```python
from build123d import *

# Parameters (mm, degrees)
BOSS_EXTRUDE1_DEPTH = 50.8
SKETCH2_R           = 2.667
CUT_EXTRUDE1_DEPTH  = 3.175
SKETCH3_R           = 2.667
CUT_EXTRUDE2_DEPTH  = 3.175
FILLET1_R           = 2.159


with BuildPart() as part:
    # Sketch1 → Boss-Extrude1 (new body)
    with BuildSketch(Plane(origin=(0, 0, 0), x_dir=(0, 0, -1), z_dir=(1, 0, 0))):
        Polygon((0, 0), (0, 25.4), (-3.175, 25.4), (-3.175, 3.175), (-25.4, 3.175), (-25.4, 0), align=None)
    extrude(amount=BOSS_EXTRUDE1_DEPTH)

    # Sketch2 → Cut-Extrude1 (cut)
    with BuildSketch(Plane(origin=(0, 3.175, 0), x_dir=(1, 0, 0), z_dir=(0, 1, 0))):
        with Locations((11.938, -19.05)):
            Circle(SKETCH2_R)
        with Locations((37.338, -19.05)):
            Circle(SKETCH2_R)
    extrude(amount=-CUT_EXTRUDE1_DEPTH, mode=Mode.SUBTRACT)

    # Sketch3 → Cut-Extrude2 (cut)
    with BuildSketch(Plane.XY.offset(3.175)):
        with Locations((38.1, 14.351)):
            Circle(SKETCH3_R)
        with Locations((12.7, 14.351)):
            Circle(SKETCH3_R)
    extrude(amount=-CUT_EXTRUDE2_DEPTH, mode=Mode.SUBTRACT)

    # Fillet1
    fillet1_edges = [part.edges().sort_by_distance(p)[0] for p in [
        (25.4, 3.175, 3.175),
        (25.4, 0, 0),
    ]]
    fillet(fillet1_edges, radius=FILLET1_R)


solid = part.part
```
Geometry: final body of the model. Coordinates: model frame, mm. A direction names the side the tool comes from. Round coordinates to 2 decimals unless told otherwise and drop trailing zeros. Loops run counter-clockwise (first coordinate to the right, second up) from the corner with the lowest first, then second, coordinate; pieces in that order, holes last.
Item 1: Mould query, pull axis Y, two halves, no side actions, for faces 1 (the flat face through (0, 2, 6)), 2 (the flat face through (25, 0, 14)), 3 (the cylindrical face through (36.13, 16.15, 1.61)). Classes: released by +Y, released by -Y, zero draft, split by the parting line, or undercut.
Checked values:
face 1: zero draft
face 2: released by -Y
face 3: undercut
Item 2: Contact query for flat-ended pins moving along their axis: P1, Ø5, axis at x = 12.7, y = 14.351, coming from the -Z side; P2, Ø8.5, axis at x = 37.338, z = 19.05, coming from the +Y side (3 decimals); P3, Ø5, axis at x = 38.5, y = 17, coming from the +Z side (3 decimals). Output: stop coordinate, or through.
Checked values:
P1: passes through
P2: stops at y = 3.175
P3: stops at z = 3.175
Item 3: Section A-A, the plane z = 19.05. Output: boundary loops of the cut face in (x, y) (3 decimals).
Checked values:
outline: (0, 0) - (9.271, 0) - (9.271, 3.175) - (0, 3.175) - close; (14.605, 0) - (34.671, 0) - (34.671, 3.175) - (14.605, 3.175) - close; (40.005, 0) - (50.8, 0) - (50.8, 3.175) - (40.005, 3.175) - close
Item 4: Section D-D, the plane x = 25.5. Output: boundary loops of the cut face in (y, z) (3 decimals).
Checked values:
outline: (0, 2.159) arc R2.159 ccw to (2.159, 0) - (25.4, 0) - (25.4, 3.175) - (5.334, 3.175) arc R2.159 cw to (3.175, 5.334) - (3.175, 25.4) - (0, 25.4) - close
Item 5: Section C-C, the plane x = 38.1. Output: boundary loops of the cut face in (y, z) (3 decimals), plus the area to 3 significant figures.
Checked values:
outline: (0, 2.159) arc R2.159 ccw to (2.159, 0) - (11.684, 0) - (11.684, 3.175) - (5.334, 3.175) arc R2.159 cw to (3.175, 5.334) - (3.175, 16.494) - (0, 16.494) - close; (0, 21.606) - (3.175, 21.606) - (3.175, 25.4) - (0, 25.4) - close; (17.018, 0) - (25.4, 0) - (25.4, 3.175) - (17.018, 3.175) - close
area: 118 mm2
Item 6: Line query: L1, parallel to X at y = 2.25, z = 19.05 (3 decimals); L2, parallel to Y at x = 22, z = 5.25; L3, parallel to Z at x = 42, y = 10.5 (3 decimals). Output: solid intervals per line, ascending.
Checked values:
L1: x = 0 to 9.271, 14.605 to 34.671, 40.005 to 50.8
L2: y = 0 to 3.18
L3: z = 0 to 3.175
Item 7: Section B-B, the plane y = 16. Output: boundary loops of the cut face in (x, z) (3 decimals), plus the area to 3 significant figures.
Checked values:
outline: (0, 0) - (10.604, 0) - (10.604, 3.175) - (0, 3.175) - close; (14.796, 0) - (36.004, 0) - (36.004, 3.175) - (14.796, 3.175) - close; (40.196, 0) - (50.8, 0) - (50.8, 3.175) - (40.196, 3.175) - close
area: 135 mm2
Item 8: Reachability of faces 4 (the flat face through (25, 25.4, 2)), 5 (the flat face through (25, 16, 3.175)) from +Z, -Z, +X, -X, +Y, -Y: full face, straight path, thin tool, end or side. Return the list, or none.
Checked values:
face 4: +Z, -Z, +X, -X, +Y
face 5: +Z, +X, -X, +Y
